Read the model definition and answer for the solid it produces. Units are mm, in the model's axes. Give positions to 0.01 mm unless a question says otherwise; leave off trailing zeros. Write each loop counter-clockwise with the first axis right and the second up, starting at its lowest first coordinate (ties: lowest second). Pieces come first, ordered by that corner, then holes. Notation, with made-up numbers: (68.5, -2) -> (72.5, -2) arc R14 cw to (72.5, 10) -> close; hole circle Ø11 at (21.25, 17). An arc over 180 degrees is marked (long way). Write item = value, one per line.
from build123d import *

# Parameters (mm, degrees)
SKETCH1_W           = 152.4
SKETCH1_H           = 88.9
BOSS_EXTRUDE1_DEPTH = 3.175
SKETCH2_W           = 3.175
SKETCH2_H           = 44.45
CUT_EXTRUDE1_DEPTH  = 4.175
SKETCH3_R           = 1.8288
CUT_EXTRUDE2_DEPTH  = 4.175
SKETCH6_W           = 3.175
SKETCH6_H           = 25.4
BOSS_EXTRUDE2_DEPTH = 3.175
CUT_EXTRUDE3_DEPTH  = 4.175
CUT_EXTRUDE4_DEPTH  = 4.175
SKETCH9_W           = 152.4
SKETCH9_H           = 20.955
BOSS_EXTRUDE3_DEPTH = 3.175
SKETCH10_R          = 1.8288
CUT_EXTRUDE5_DEPTH  = 4.175
SKETCH11_W          = 120.142
SKETCH11_H          = 88.9
BOSS_EXTRUDE4_DEPTH = 3.175
SKETCH12_R          = 6.35
CUT_EXTRUDE6_DEPTH  = 4.175
SKETCH13_R          = 1.8288
CUT_EXTRUDE7_DEPTH  = 4.175
SKETCH14_R          = 1.8288
CUT_EXTRUDE8_DEPTH  = 101.6
SKETCH15_R          = 1.8288
CUT_EXTRUDE9_DEPTH  = 4.175


with BuildPart() as part:
    # Sketch1 → Boss-Extrude1 (new body)
    with BuildSketch(Plane(origin=(0, 0, 0), x_dir=(1, 0, 0), z_dir=(0, 1, 0))):
        Rectangle(SKETCH1_W, SKETCH1_H)
    extrude(amount=BOSS_EXTRUDE1_DEPTH)

    # Sketch2 → Cut-Extrude1 (cut, through all)
    with BuildSketch(Plane(origin=(0, 3.175, 0), x_dir=(1, 0, 0), z_dir=(0, 1, 0))):
        with Locations((61.9125, 22.225)):
            Rectangle(SKETCH2_W, SKETCH2_H)
        with Locations((-61.9125, 22.225)):
            Rectangle(SKETCH2_W, SKETCH2_H)
    extrude(amount=-CUT_EXTRUDE1_DEPTH, mode=Mode.SUBTRACT)

    # Sketch3 → Cut-Extrude2 (cut, through all)
    with BuildSketch(Plane(origin=(0, 3.175, 0), x_dir=(1, 0, 0), z_dir=(0, 1, 0))):
        with Locations((-70.993, -25.4)):
            Circle(SKETCH3_R)
        with Locations((-70.993, 0)):
            Circle(SKETCH3_R)
        with Locations((-70.993, 25.4)):
            Circle(SKETCH3_R)
        with Locations((70.993, -25.4)):
            Circle(SKETCH3_R)
        with Locations((70.993, 0)):
            Circle(SKETCH3_R)
        with Locations((70.993, 25.4)):
            Circle(SKETCH3_R)
    extrude(amount=-CUT_EXTRUDE2_DEPTH, mode=Mode.SUBTRACT)

    # Sketch6 → Boss-Extrude2 (add)
    with BuildSketch(Plane(origin=(0, 3.175, 0), x_dir=(1, 0, 0), z_dir=(0, 1, 0))):
        with Locations((-61.9125, 12.7)):
            Rectangle(SKETCH6_W, SKETCH6_H)
        with Locations((61.9125, 12.7)):
            Rectangle(SKETCH6_W, SKETCH6_H)
    extrude(amount=-BOSS_EXTRUDE2_DEPTH)

    # Sketch7 → Cut-Extrude3 (cut, through all)
    with BuildSketch(Plane(origin=(0, 3.175, 0), x_dir=(1, 0, 0), z_dir=(0, 1, 0))):
        Polygon((-63.754, 44.45), (-63.5, 44.45), (-63.5, 25.4), (-60.325, 25.4), (-60.325, 44.45), (-60.071, 44.45), (-60.071, 25.146), (-63.754, 25.146), align=None)
    extrude(amount=-CUT_EXTRUDE3_DEPTH, mode=Mode.SUBTRACT)

    # Sketch8 → Cut-Extrude4 (cut, through all)
    with BuildSketch(Plane(origin=(0, 3.175, 0), x_dir=(1, 0, 0), z_dir=(0, 1, 0))):
        Polygon((60.071, 44.45), (60.325, 44.45), (60.325, 25.4), (63.5, 25.4), (63.5, 44.45), (63.754, 44.45), (63.754, 25.146), (60.071, 25.146), align=None)
    extrude(amount=-CUT_EXTRUDE4_DEPTH, mode=Mode.SUBTRACT)

    # Sketch9 → Boss-Extrude3 (add)
    with BuildSketch(Plane(origin=(0, 3.175, 0), x_dir=(1, 0, 0), z_dir=(0, 1, 0))):
        with Locations((0, -54.9275)):
            Rectangle(SKETCH9_W, SKETCH9_H)
    extrude(amount=-BOSS_EXTRUDE3_DEPTH)

    # Sketch10 → Cut-Extrude5 (cut, through all)
    with BuildSketch(Plane(origin=(0, 3.175, 0), x_dir=(1, 0, 0), z_dir=(0, 1, 0))):
        with Locations((-73.1647, -57.531)):
            Circle(SKETCH10_R)
        with Locations((-46.2153, -57.531)):
            Circle(SKETCH10_R)
        with Locations((46.2153, -57.531)):
            Circle(SKETCH10_R)
        with Locations((73.1647, -57.531)):
            Circle(SKETCH10_R)
    extrude(amount=-CUT_EXTRUDE5_DEPTH, mode=Mode.SUBTRACT)

    # Sketch11 → Boss-Extrude4 (add)
    with BuildSketch(Plane(origin=(0, 3.175, 0), x_dir=(1, 0, 0), z_dir=(0, 1, 0))):
        with Locations((0, 33.02)):
            Rectangle(SKETCH11_W, SKETCH11_H)
    extrude(amount=-BOSS_EXTRUDE4_DEPTH)

    # Sketch12 → Cut-Extrude6 (cut, through all)
    with BuildSketch(Plane(origin=(0, 3.175, 0), x_dir=(1, 0, 0), z_dir=(0, 1, 0))):
        with Locations((0, 33.02)):
            Circle(SKETCH12_R)
    extrude(amount=-CUT_EXTRUDE6_DEPTH, mode=Mode.SUBTRACT)

    # Sketch13 → Cut-Extrude7 (cut, through all)
    with BuildSketch(Plane(origin=(0, 3.175, 0), x_dir=(1, 0, 0), z_dir=(0, 1, 0))):
        with Locations((32.5501, 0.4699)):
            Circle(SKETCH13_R)
        with Locations((-32.5501, 0.4699)):
            Circle(SKETCH13_R)
        with Locations((-32.5501, 65.5701)):
            Circle(SKETCH13_R)
        with Locations((32.5501, 65.5701)):
            Circle(SKETCH13_R)
    extrude(amount=-CUT_EXTRUDE7_DEPTH, mode=Mode.SUBTRACT)

    # Sketch14 → Cut-Extrude8 (cut)
    with BuildSketch(Plane.XZ):
        with Locations((0, -23.241)):
            Circle(SKETCH14_R)
        with Locations((-9.779, -33.02)):
            Circle(SKETCH14_R)
        with Locations((0, -42.799)):
            Circle(SKETCH14_R)
        with Locations((9.779, -33.02)):
            Circle(SKETCH14_R)
    extrude(amount=-CUT_EXTRUDE8_DEPTH, mode=Mode.SUBTRACT)

    # Sketch15 → Cut-Extrude9 (cut, through all)
    with BuildSketch(Plane.XZ):
        with Locations((-42.291, 26.162)):
            Circle(SKETCH15_R)
        with Locations((-42.291, -0.7874)):
            Circle(SKETCH15_R)
    extrude(amount=-CUT_EXTRUDE9_DEPTH, mode=Mode.SUBTRACT)


solid = part.part
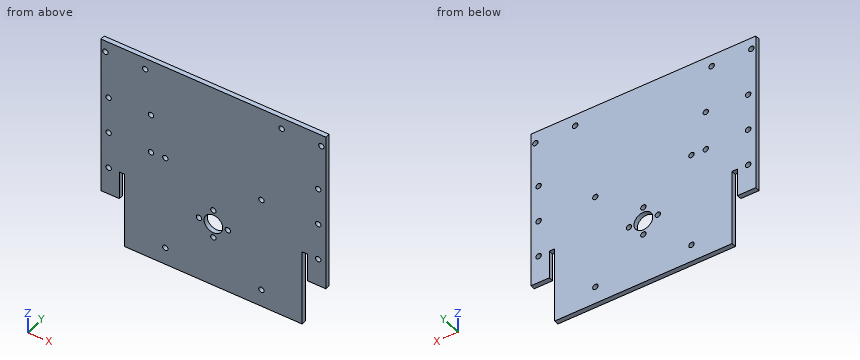
(1) Consider L1, parallel to X at y = 2.55, z = -25.4; L2, parallel to X at y = 1.8, z = 25.5; L3, parallel to Z at x = 69.5, y = 2.8 (3 decimals). Determine where each line is inside the solid, lowest interval first.
Checks:
L1 = -76.2 to -72.82, -69.16 to -63.75, -60.07 to 60.07, 63.75 to 69.16, 72.82 to 76.2
L2 = -76.2 to -72.82, -69.17 to -44, -40.59 to 69.17, 72.82 to 76.2
L3 = -44.45 to -26.456, -24.344 to -1.056, 1.056 to 24.344, 26.456 to 65.405
(2) Given P1, Ø3, axis at x = -32.55, z = -0.47, coming from the -Y side; P2, Ø1.6, axis at y = 1, z = -56, coming from the +X side, each flat-ended and moving along its own axis, determine where each tip first touches the part or whether it passes through.
Checks:
P1 = through
P2 = 60.07
(3) The part is cut by section B-B on x = 0. Determine the outline of the cut face in (y, z) (3 decimals).
Checks:
outline = (0, -77.47) -> (3.175, -77.47) -> (3.175, -44.628) -> (0, -44.628) -> close; (0, -40.97) -> (3.175, -40.97) -> (3.175, -39.37) -> (0, -39.37) -> close; (0, -26.67) -> (3.175, -26.67) -> (3.175, -25.07) -> (0, -25.07) -> close; (0, -21.412) -> (3.175, -21.412) -> (3.175, 65.405) -> (0, 65.405) -> close
(4) The part is cut by section C-C on y = 0.5. Count the separate pieces of the cut face and the enclosed holes in it, plus the area to 3 significant figures.
Checks:
separate_pieces = 1
enclosed_holes = 21
area = 20,200 mm²
(5) The part is cut by section A-A on z = -33.02. Determine the outline of the cut face in (x, y) (3 decimals).
Checks:
outline = (-76.2, 0) -> (-63.754, 0) -> (-63.754, 3.175) -> (-76.2, 3.175) -> close; (-60.071, 0) -> (-11.608, 0) -> (-11.608, 3.175) -> (-60.071, 3.175) -> close; (-7.95, 0) -> (-6.35, 0) -> (-6.35, 3.175) -> (-7.95, 3.175) -> close; (6.35, 0) -> (7.95, 0) -> (7.95, 3.175) -> (6.35, 3.175) -> close; (11.608, 0) -> (60.071, 0) -> (60.071, 3.175) -> (11.608, 3.175) -> close; (63.754, 0) -> (76.2, 0) -> (76.2, 3.175) -> (63.754, 3.175) -> close
